from build123d import *

# Parameters (mm, degrees)
F0_W     = 95.7474842701
F0_H     = 77.4886654093
F0_R     = 15
F1_DEPTH = 40
F2_W     = 95.7474842701
F2_H     = 20
F3_DEPTH = 40
F4_R     = 6.3464300443
F5_DEPTH = 25


# Not quite as in the source:
# - a pattern or mirror of a feature is missing from the dataset's text; its kind, count and spacing are read off the source's solid


with BuildPart() as f1:
    # F0 (on Top) → F1 (new body)
    with BuildSketch(Plane.XY):
        with Locations((0.8906734218, -2.0040220562)):
            Rectangle(F0_W, F0_H)
        Circle(F0_R, mode=Mode.SUBTRACT)
    extrude(amount=F1_DEPTH)

    # F2 (on face) → F3 (cut)
    with BuildSketch(Plane.XZ.offset(40.7483547609)):
        with Locations((0.8906734218, 17.9856412485)):
            Rectangle(F2_W, F2_H)
    extrude(amount=-F3_DEPTH, mode=Mode.SUBTRACT)

    # F4 (on face) → F5 (cut)
    with BuildSketch(Plane(origin=(0, 0, 0), x_dir=(1, 0, 0), z_dir=(0, 0, -1))):
        with Locations((23.8608885556, 26.9455648959)):
            Circle(F4_R)
    f5 = extrude(amount=-F5_DEPTH, mode=Mode.SUBTRACT)

    # F5_copies: F5 across plane
    add(f5.mirror(Plane(origin=(0, 0, 0), x_dir=(0, 0, -1), z_dir=(-1, 0, 0))), mode=Mode.SUBTRACT)


solid = f1.part
Can you work these out from the model? Positions are in its coordinate system, mm. A direction names the side the tool comes from. Give positions to 0.01 mm unless a question says otherwise; leave off trailing zeros. Order: outer loops, then holes, each group sorted by start corner. A loop starts at its lowest first (then second) coordinate and runs counter-clockwise, first axis right, second up. Notation, with made-up numbers: M -29,66.5 L -2,66.5 A29 cw -2,97.5 Z; hole C 35,-4 d7. An arc over 180 degrees is marked long. One line per item, written item: value.
Item 1: If we section it at B-B on z = 36: Write out the boundary of the cut face in (x, y), and give its area (3 significant figures).
Verdict:
outline: M -46.98,-40.75 L 48.76,-40.75 L 48.76,36.74 L -46.98,36.74 Z; hole C 0,0 d30
area: 6,710 mm2
Item 2: For faces 1 (the face through (48.764, 6, 20)), 2 (the face through (32, -0.748, 18)), 3 (the face through (-22.49, -20.75, 3.94)), which set-ups out of +Z, -Z, +X, -X, +Y, -Y let a thin tool reach every point of the face, with its end or its side?
Verdict:
face 1: +Z, -Z, +X, +Y, -Y
face 2: +X, -X, -Y
face 3: -Z
Item 3: For pin 1 (10 mm diameter, centred on x = -28.5, z = 20.5, fed in from -Y); pin 2 (18 mm diameter, centred on x = 0, y = 0, fed in from +Z), each with a flat end and sliding along its axis, tell me the tip position at first contact or that it passes through.
Verdict:
pin 1: y = -0.75
pin 2: through
Item 4: Please list where these lines run through material, in increasing order: line 1 (Z direction, x = 10, y = -23); line 2 (Y direction, x = 0, z = 11); line 3 (Y direction, x = 21, z = 13).
Verdict:
line 1: 0 to 7.99, 27.99 to 40
line 2: 15 to 36.74
line 3: -0.75 to 36.74
Item 5: If we section it at A-A on x = 0: Write out the boundary of the cut face in (y, z).
Verdict:
outline: M -40.75,0 L -15,0 L -15,7.99 L -40.75,7.99 Z; M -40.75,27.99 L -15,27.99 L -15,40 L -40.75,40 Z; M 15,0 L 36.74,0 L 36.74,40 L 15,40 Z
Item 6: If we mould it in two halves opening along Z, with no side actions, what happens to faces 4 (the face through (0, 36.74, 20)), 5 (the face through (-31, -0.748, 18)), 6 (the face through (0, 16, 40))? For each: pulls with the +Z half, pulls with the -Z half, needs draft (parallel to the pull), parting line crosses it, or undercut.
Verdict:
face 4: needs draft
face 5: undercut
face 6: pulls with the +Z half
Item 7: If we section it at C-C on x = 24: Write out the boundary of the cut face in (y, z), and give its area (3 significant figures).
Verdict:
outline: M -40.75,0 L -33.29,0 L -33.29,7.99 L -40.75,7.99 Z; M -40.75,27.99 L -0.75,27.99 L -0.75,7.99 L -20.6,7.99 L -20.6,0 L 36.74,0 L 36.74,40 L -40.75,40 Z
area: 2,200 mm2
Item 8: If we section it at D-D on x = -33.5: Write out the boundary of the cut face in (y, z), and give its area (3 significant figures).
Verdict:
outline: M -40.75,0 L 36.74,0 L 36.74,40 L -40.75,40 L -40.75,27.99 L -0.75,27.99 L -0.75,7.99 L -40.75,7.99 Z
area: 2,300 mm2
